from build123d import *

# Parameters (mm, degrees)
SKETCH2_W            = 80
SKETCH2_H            = 40
BOSS_EXTRUDE2_DEPTH  = 10
SKETCH3_R            = 5
CUT_EXTRUDE1_DEPTH   = 11
LPATTERN2_COUNT      = 4
LPATTERN2_PITCH      = 20
LPATTERN2_COUNT_DIR2 = 2
LPATTERN2_PITCH_DIR2 = 20
FILLET1_R            = 2


with BuildPart() as part:
    # Sketch2 → Boss-Extrude2 (new body)
    with BuildSketch(Plane.XY):
        with Locations((40, 20)):
            Rectangle(SKETCH2_W, SKETCH2_H)
    extrude(amount=BOSS_EXTRUDE2_DEPTH)

    # Sketch3 → Cut-Extrude1 (cut, through all)
    with BuildSketch(Plane.XY.offset(10)):
        with Locations((10, 10)):
            Circle(SKETCH3_R)
    cut_extrude1 = extrude(amount=-CUT_EXTRUDE1_DEPTH, mode=Mode.SUBTRACT)

    # LPattern2: Cut-Extrude1 4 × 2
    with Locations(*[(i * LPATTERN2_PITCH, j * LPATTERN2_PITCH_DIR2, 0) for i in range(LPATTERN2_COUNT) for j in range(LPATTERN2_COUNT_DIR2) if (i, j) != (0, 0)]):
        add(cut_extrude1, mode=Mode.SUBTRACT)

    # Fillet1
    fillet1_edges = [part.edges().sort_by_distance(p)[0] for p in [
        (0, 40, 5),
        (80, 40, 5),
        (80, 0, 5),
        (0, 0, 5),
    ]]
    fillet(fillet1_edges, radius=FILLET1_R)


solid = part.part
Geometry: final body of the model. Coordinates: model frame, mm. Round coordinates to 2 decimals unless told otherwise and drop trailing zeros. Loops run counter-clockwise (first coordinate to the right, second up) from the corner with the lowest first, then second, coordinate; pieces in that order, holes last.
Q1. Section B-B on x = 10. Return loops of the section in (y, z), plus the area to 3 significant figures.
Q2. Section A-A on y = 30. Return loops of the section in (x, z), plus the area to 3 significant figures.
Q3. Pull-direction query (X, two-part tool) for faces 1 (the cylindrical face through (14.77, 11.5, 5.07)), 2 (the cylindrical face through (79.4, 39.43, 5.07)), 3 (the cylindrical face through (0.57, 0.6, 5.07)); classes: released by +X, released by -X, zero draft, split by the parting line, or undercut.
Q4. Section C-C on z = 3. State how many separate pieces and enclosed holes the cut face has, plus the area to 3 significant figures.
Q5. Material intervals for L1, parallel to Y at x = 70, z = 5.25; L2, parallel to X at y = 8, z = 1.75; L3, parallel to Y at x = 26, z = 5.5, sorted ascending.
Q6. Pin query (flat end, axial travel): P1, Ø6, axis at x = 71, y = 21.5, coming from the -Z side. Return the tip coordinate at first contact, or that it passes through.
Q7. Section D-D on y = 14. Return loops of the section in (x, z).
Evaluation:
1. outline: (0, 0) - (5, 0) - (5, 10) - (0, 10) - close; (15, 0) - (25, 0) - (25, 10) - (15, 10) - close; (35, 0) - (40, 0) - (40, 10) - (35, 10) - close
1. area: 200 mm2
2. outline: (0, 0) - (5, 0) - (5, 10) - (0, 10) - close; (15, 0) - (25, 0) - (25, 10) - (15, 10) - close; (35, 0) - (45, 0) - (45, 10) - (35, 10) - close; (55, 0) - (65, 0) - (65, 10) - (55, 10) - close; (75, 0) - (80, 0) - (80, 10) - (75, 10) - close
2. area: 400 mm2
3. face 1: undercut
3. face 2: released by +X
3. face 3: released by -X
4. separate pieces: 1
4. enclosed holes: 8
4. area: 2,570 mm2
5. L1: y = 0 to 5, 15 to 25, 35 to 40
5. L2: x = 0 to 5.42, 14.58 to 25.42, 34.58 to 45.42, 54.58 to 65.42, 74.58 to 80
5. L3: y = 0 to 7, 13 to 27, 33 to 40
6. P1: stops at z = 0
7. outline: (0, 0) - (7, 0) - (7, 10) - (0, 10) - close; (13, 0) - (27, 0) - (27, 10) - (13, 10) - close; (33, 0) - (47, 0) - (47, 10) - (33, 10) - close; (53, 0) - (67, 0) - (67, 10) - (53, 10) - close; (73, 0) - (80, 0) - (80, 10) - (73, 10) - close
